from build123d import *

# Parameters (mm, degrees)
SKETCH1_W           = 260
SKETCH1_H           = 270
BOSS_EXTRUDE1_DEPTH = 6
SKETCH2_W           = 20
SKETCH2_H           = 6
CUT_EXTRUDE1_DEPTH  = 6
SKETCH4_W           = 6
SKETCH4_H           = 44.5
SKETCH4_H_2         = 15
SKETCH4_H_3         = 36
CUT_EXTRUDE3_DEPTH  = 6
SKETCH5_R           = 8
CUT_EXTRUDE4_DEPTH  = 10
SKETCH6_R           = 8
SKETCH6_R_2         = 1.55
CUT_EXTRUDE5_DEPTH  = 6
SKETCH7_R           = 1.55
CUT_EXTRUDE6_DEPTH  = 10
SKETCH8_W           = 248
SKETCH8_H           = 6
BOSS_EXTRUDE2_DEPTH = 5
SKETCH9_W           = 4.5
SKETCH9_H           = 275
BOSS_EXTRUDE5_DEPTH = 6
SKETCH10_R          = 13.75
CUT_EXTRUDE7_DEPTH  = 6
SKETCH11_R          = 1.55
CUT_EXTRUDE8_DEPTH  = 6
SKETCH12_R          = 1.55
CUT_EXTRUDE9_DEPTH  = 10
SKETCH13_W          = 44.5
SKETCH13_H          = 6
BOSS_EXTRUDE6_DEPTH = 4
SKETCH14_W          = 269
SKETCH14_H          = 6
BOSS_EXTRUDE7_DEPTH = 14
SKETCH15_R          = 1.55
SKETCH15_W          = 20
SKETCH15_H          = 6
CUT_EXTRUDE10_DEPTH = 10
SKETCH16_R          = 1.25
CUT_EXTRUDE11_DEPTH = 10


with BuildPart() as part:
    # Sketch1 → Boss-Extrude1 (new body)
    with BuildSketch(Plane.XY):
        with Locations((130, 135)):
            Rectangle(SKETCH1_W, SKETCH1_H)
    extrude(amount=BOSS_EXTRUDE1_DEPTH)

    # Sketch2 → Cut-Extrude1 (cut)
    with BuildSketch(Plane(origin=(0, 0, 0), x_dir=(-1, 0, 0), z_dir=(0, 0, -1))):
        with Locations((-215, 53)):
            Rectangle(SKETCH2_W, SKETCH2_H)
        with Locations((-175, 53)):
            Rectangle(SKETCH2_W, SKETCH2_H)
        with BuildLine():
            Line((-220, 0), (-40, 0))
            ThreePointArc((-40, 0), (-130, 10), (-220, 0))
        make_face()
        with Locations((-85, 53)):
            Rectangle(SKETCH2_W, SKETCH2_H)
        with Locations((-45, 53)):
            Rectangle(SKETCH2_W, SKETCH2_H)
    extrude(amount=-CUT_EXTRUDE1_DEPTH, mode=Mode.SUBTRACT)

    # Sketch4 → Cut-Extrude3 (cut)
    with BuildSketch(Plane(origin=(0, 0, 0), x_dir=(-1, 0, 0), z_dir=(0, 0, -1))):
        Polygon((-254, 270), (-260, 270), (-260, 264), (-260, 255), (-254, 255), (-254, 264), align=None)
        with Locations((-257, 212.75)):
            Rectangle(SKETCH4_W, SKETCH4_H)
        with Locations((-257, 163)):
            Rectangle(SKETCH4_W, SKETCH4_H_2)
        with Locations((-257, 113.25)):
            Rectangle(SKETCH4_W, SKETCH4_H)
        with Locations((-257, 53)):
            Rectangle(SKETCH4_W, SKETCH4_H_3)
        with Locations((-257, 7.5)):
            Rectangle(SKETCH4_W, SKETCH4_H_2)
        with Locations((-3, 7.5)):
            Rectangle(SKETCH4_W, SKETCH4_H_2)
        with Locations((-3, 53)):
            Rectangle(SKETCH4_W, SKETCH4_H_3)
        with Locations((-3, 113.25)):
            Rectangle(SKETCH4_W, SKETCH4_H)
        with Locations((-3, 212.75)):
            Rectangle(SKETCH4_W, SKETCH4_H)
        with Locations((-3, 262.5)):
            Rectangle(SKETCH4_W, SKETCH4_H_2)
        with Locations((-3, 163)):
            Rectangle(SKETCH4_W, SKETCH4_H_2)
    extrude(amount=-CUT_EXTRUDE3_DEPTH, mode=Mode.SUBTRACT)

    # Sketch5 → Cut-Extrude4 (cut)
    with BuildSketch(Plane(origin=(0, 0, 0), x_dir=(-1, 0, 0), z_dir=(0, 0, -1))):
        with Locations((-235, 240.5)):
            Circle(SKETCH5_R)
        with Locations((-25, 240.5)):
            Circle(SKETCH5_R)
    extrude(amount=-CUT_EXTRUDE4_DEPTH, mode=Mode.SUBTRACT)

    # Sketch6 → Cut-Extrude5 (cut)
    with BuildSketch(Plane(origin=(0, 0, 0), x_dir=(-1, 0, 0), z_dir=(0, 0, -1))):
        with Locations((-235, 240.5)):
            Circle(SKETCH6_R)
        with Locations((-248, 240.5)):
            Circle(SKETCH6_R_2)
        with Locations(Location((-222, 240.5, 0), (0, 0, 180))):
            Circle(SKETCH6_R_2)
        with Locations(Location((-12, 240.5, 0), (0, 0, 180))):
            Circle(SKETCH6_R_2)
        with Locations((-38, 240.5)):
            Circle(SKETCH6_R_2)
    extrude(amount=-CUT_EXTRUDE5_DEPTH, mode=Mode.SUBTRACT)

    # Sketch7 → Cut-Extrude6 (cut)
    with BuildSketch(Plane(origin=(0, 0, 0), x_dir=(-1, 0, 0), z_dir=(0, 0, -1))):
        with Locations((-186.5, 205)):
            Circle(SKETCH7_R)
        with Locations((-148.9, 205)):
            Circle(SKETCH7_R)
        with Locations((-148.9, 219)):
            Circle(SKETCH7_R)
        with Locations((-186.5, 219)):
            Circle(SKETCH7_R)
        with Locations((-73.5, 205)):
            Circle(SKETCH7_R)
        with Locations((-111.1, 205)):
            Circle(SKETCH7_R)
        with Locations((-111.1, 219)):
            Circle(SKETCH7_R)
        with Locations((-73.5, 219)):
            Circle(SKETCH7_R)
    extrude(amount=-CUT_EXTRUDE6_DEPTH, mode=Mode.SUBTRACT)

    # Sketch8 → Boss-Extrude2 (add)
    with BuildSketch(Plane(origin=(0, 270, 0), x_dir=(1, 0, 0), z_dir=(0, 1, 0))):
        with Locations((130, -3)):
            Rectangle(SKETCH8_W, SKETCH8_H)
    extrude(amount=BOSS_EXTRUDE2_DEPTH)

    # Sketch9 → Boss-Extrude5 (add)
    with BuildSketch(Plane(origin=(0, 0, 0), x_dir=(-1, 0, 0), z_dir=(0, 0, -1))):
        with Locations((2.25, 137.5)):
            Rectangle(SKETCH9_W, SKETCH9_H)
        with Locations((-262.25, 137.5)):
            Rectangle(SKETCH9_W, SKETCH9_H)
    extrude(amount=-BOSS_EXTRUDE5_DEPTH)

    # Sketch10 → Cut-Extrude7 (cut)
    with BuildSketch(Plane.XY.offset(6)):
        with Locations((226, 210.052298937)):
            Circle(SKETCH10_R)
        with BuildLine():
            Line((208.95, 224.052298937), (208.95, 227.052298937))
            ThreePointArc((208.95, 227.052298937), (210.5, 228.602298937), (212.05, 227.052298937))
            Line((212.05, 227.052298937), (212.05, 224.052298937))
            ThreePointArc((212.05, 224.052298937), (210.5, 222.502298937), (208.95, 224.052298937))
        make_face()
        with BuildLine():
            Line((243.05, 224.052298937), (243.05, 227.052298937))
            ThreePointArc((243.05, 227.052298937), (241.5, 228.602298937), (239.95, 227.052298937))
            Line((239.95, 227.052298937), (239.95, 224.052298937))
            ThreePointArc((239.95, 224.052298937), (241.5, 222.502298937), (243.05, 224.052298937))
        make_face()
        with BuildLine():
            Line((243.05, 193.052298937), (243.05, 196.052298937))
            ThreePointArc((243.05, 196.052298937), (241.5, 197.602298937), (239.95, 196.052298937))
            Line((239.95, 196.052298937), (239.95, 193.052298937))
            ThreePointArc((239.95, 193.052298937), (241.5, 191.502298937), (243.05, 193.052298937))
        make_face()
        with BuildLine():
            Line((212.05, 193.052298937), (212.05, 196.052298937))
            ThreePointArc((212.05, 196.052298937), (210.5, 197.602298937), (208.95, 196.052298937))
            Line((208.95, 196.052298937), (208.95, 193.052298937))
            ThreePointArc((208.95, 193.052298937), (210.5, 191.502298937), (212.05, 193.052298937))
        make_face()
    extrude(amount=-CUT_EXTRUDE7_DEPTH, mode=Mode.SUBTRACT)

    # Sketch11 → Cut-Extrude8 (cut)
    with BuildSketch(Plane.XY.offset(6)):
        with Locations((3, 245)):
            Circle(SKETCH11_R)
        with Locations((3, 180.5)):
            Circle(SKETCH11_R)
        with Locations((3, 145.5)):
            Circle(SKETCH11_R)
        with Locations((3, 81)):
            Circle(SKETCH11_R)
        with Locations((3, 25)):
            Circle(SKETCH11_R)
        with Locations(Location((257, 25, 0), (0, 0, 180))):
            Circle(SKETCH11_R)
        with Locations(Location((257, 81, 0), (0, 0, 180))):
            Circle(SKETCH11_R)
        with Locations(Location((257, 145.5, 0), (0, 0, 180))):
            Circle(SKETCH11_R)
        with Locations(Location((257, 180.5, 0), (0, 0, 180))):
            Circle(SKETCH11_R)
        with Locations(Location((257, 245, 0), (0, 0, 180))):
            Circle(SKETCH11_R)
    extrude(amount=-CUT_EXTRUDE8_DEPTH, mode=Mode.SUBTRACT)

    # Sketch12 → Cut-Extrude9 (cut)
    with BuildSketch(Plane.XY.offset(6)):
        with Locations((25, 53)):
            Circle(SKETCH12_R)
        with Locations((65, 53)):
            Circle(SKETCH12_R)
        with Locations((105, 53)):
            Circle(SKETCH12_R)
        with Locations(Location((155, 53, 0), (0, 0, 180))):
            Circle(SKETCH12_R)
        with Locations(Location((195, 53, 0), (0, 0, 180))):
            Circle(SKETCH12_R)
        with Locations(Location((235, 53, 0), (0, 0, 180))):
            Circle(SKETCH12_R)
    extrude(amount=-CUT_EXTRUDE9_DEPTH, mode=Mode.SUBTRACT)

    # Sketch13 → Boss-Extrude6 (add)
    with BuildSketch(Plane.XZ):
        with Locations((17.75, 3)):
            Rectangle(SKETCH13_W, SKETCH13_H)
        with Locations((242.25, 3)):
            Rectangle(SKETCH13_W, SKETCH13_H)
    extrude(amount=BOSS_EXTRUDE6_DEPTH)

    # Sketch14 → Boss-Extrude7 (add)
    with BuildSketch(Plane(origin=(0, 275, 0), x_dir=(1, 0, 0), z_dir=(0, 1, 0))):
        with Locations((130, -3)):
            Rectangle(SKETCH14_W, SKETCH14_H)
    extrude(amount=BOSS_EXTRUDE7_DEPTH)

    # Sketch15 → Cut-Extrude10 (cut)
    with BuildSketch(Plane.XY.offset(6)):
        with Locations((25, 278)):
            Circle(SKETCH15_R)
        with Locations((65, 278)):
            Circle(SKETCH15_R)
        with Locations((105, 278)):
            Circle(SKETCH15_R)
        with Locations((155, 278)):
            Circle(SKETCH15_R)
        with Locations((195, 278)):
            Circle(SKETCH15_R)
        with Locations((235, 278)):
            Circle(SKETCH15_R)
        with Locations((45, 278)):
            Rectangle(SKETCH15_W, SKETCH15_H)
        with Locations((85, 278)):
            Rectangle(SKETCH15_W, SKETCH15_H)
        with Locations((175, 278)):
            Rectangle(SKETCH15_W, SKETCH15_H)
        with Locations((215, 278)):
            Rectangle(SKETCH15_W, SKETCH15_H)
    extrude(amount=-CUT_EXTRUDE10_DEPTH, mode=Mode.SUBTRACT)

    # Sketch16 → Cut-Extrude11 (cut)
    with BuildSketch(Plane.XY.offset(6)):
        with Locations((179.6, 68)):
            Circle(SKETCH16_R)
        with Locations((170, 68)):
            Circle(SKETCH16_R)
    extrude(amount=-CUT_EXTRUDE11_DEPTH, mode=Mode.SUBTRACT)


solid = part.part
For this review, take the finished solid that the model builds, in its own axes (mm). A direction names the side the tool comes from. Round coordinates to 2 decimals unless told otherwise and drop trailing zeros. Order: outer loops, then holes, each group sorted by start corner. A loop starts at its lowest first (then second) coordinate and runs counter-clockwise, first axis right, second up. Notation, with made-up numbers: M 3,-26 L 35,-26 A21 ccw 35,-12 Z; hole C -33.5,83.5 d1. An arc over 180 degrees is marked long. Write each question's results on one line, items separated by ' | '. Start each with the question number.
1. Tool access review of faces 1 (the face through (45, 56, 3)), 2 (the face through (242, -4, 3)): name each direction out of +Z, -Z, +X, -X, +Y, -Y from which nothing blocks a thin tool from reaching the whole face with its end or side.
2. Add section C-C (z = 3). State how many separate pieces and enclosed holes the cut face has, then the cut area to 3 significant figures.
3. Add section B-B (x = 49.5). State the section outline as (y, z) points.
4. Draft analysis for pull direction X (two halves, no side actions). For faces 3 (the face through (35, 53, 3)), 4 (the face through (128, 140, 0)), 5 (the face through (0, 212, 3)), 6 (the face through (-4.5, 140, 3)), state which applies: pulls with the +X half, pulls with the -X half, needs draft (parallel to the pull), parting line crosses it, or undercut.
5. To check wall thickness, follow L1, parallel to X at y = 46, z = 1.9; L2, parallel to Y at x = 167, z = 1.3; L3, parallel to X at y = 80.5, z = 3.25. State the ranges of each line that lie inside material, in increasing order. Write a range as [from, to].
6. Add section A-A (y = 101.5). State the section outline as (x, z) points, then the cut area to 3 significant figures.
7. Clearance check with a flat-ended pin moving along its axis: pin 1 Ø2 at (x, z) = (70, 2) entering from -Y. State where the tip first meets the part, or that it passes through.
8. Add section D-D (x = 128). State the section outline as (y, z) points.
Output values:
1) face 1: +Z, -Z | face 2: +Z, -Z, +X, -X, -Y
2) separate pieces: 1 | enclosed holes: 63 | area: 72,500 mm^2
3) outline: M 2.02,0 L 50,0 L 50,6 L 2.02,6 Z; M 56,0 L 275,0 L 275,6 L 56,6 Z; M 281,0 L 289,0 L 289,6 L 281,6 Z
4) face 3: undercut | face 4: needs draft | face 5: undercut | face 6: pulls with the -X half
5) L1: [-4.5, 0], [6, 254], [260, 264.5] | L2: [8.33, 50], [56, 275], [281, 289] | L3: [-4.5, 1.53], [4.47, 255.53], [258.47, 264.5]
6) outline: M -4.5,0 L 0,0 L 0,6 L -4.5,6 Z; M 6,0 L 254,0 L 254,6 L 6,6 Z; M 260,0 L 264.5,0 L 264.5,6 L 260,6 Z | area: 1,540 mm^2
7) pin 1: y = 5.44
8) outline: M 10,0 L 289,0 L 289,6 L 10,6 Z
